from build123d import *

# Parameters (mm, degrees)
BOSS_EXTRUDE1_DEPTH      = 6.35
FILLET1_R                = 12.7
CUT_EXTRUDE2_DEPTH       = 3.175
BOSS_EXTRUDE2_DEPTH      = 3.175
BOSS_EXTRUDE2_DEPTH_BACK = 36.135303
SKETCH4_R                = 9.525
SKETCH4_R_2              = 6.35
SKETCH5_R                = 9.525
SKETCH5_R_2              = 6.35
BOSS_EXTRUDE3_DEPTH      = 25.4
CHAMFER2_SIZE            = 1


with BuildPart() as part:
    # Sketch1 → Boss-Extrude1 (new, symmetric)
    with BuildSketch(Plane.YZ):
        Polygon((-25.4, 10.735303163), (0, 25.4), (25.4, 25.4), (25.4, -25.4), (-25.4, -25.4), align=None)
    extrude(amount=BOSS_EXTRUDE1_DEPTH, both=True)

    # Fillet1
    fillet1_edges = [part.edges().sort_by_distance(p)[0] for p in [
        (0, 25.4, -25.4),
    ]]
    fillet(fillet1_edges, radius=FILLET1_R)

    # Sketch3 → Cut-Extrude2 (cut)
    with BuildSketch(Plane.YZ.offset(6.35)):
        with BuildLine():
            Line((-22.225, -22.225), (12.7, -22.225))
            ThreePointArc((12.7, -22.225), (19.435192091, -19.435192091), (22.225, -12.7))
            Line((22.225, -12.7), (22.225, 22.225))
            Line((22.225, 22.225), (0.850738686, 22.225))
            Line((0.850738686, 22.225), (-22.225, 8.902216058))
            Line((-22.225, 8.902216058), (-22.225, -22.225))
        make_face()
    cut_extrude2 = extrude(amount=-CUT_EXTRUDE2_DEPTH, mode=Mode.SUBTRACT)

    # Mirror1: Cut-Extrude2 across plane
    add(cut_extrude2.mirror(Plane(origin=(0, 0, 0), x_dir=(0, 0, 1), z_dir=(1, 0, 0))), mode=Mode.SUBTRACT)

    # Sketch4 → Boss-Extrude2 (add, two sides: drawn at the far end of the back side and taken through both)
    with BuildSketch(Plane(origin=(0, 0, -25.4), x_dir=(1, 0, 0), z_dir=(0, 0, -1)).offset(-BOSS_EXTRUDE2_DEPTH_BACK)):
        with Locations(Location((0, 33.02, 0), (0, 0, 233.130102354))):
            Circle(SKETCH4_R)
        with Locations(Location((0, 33.02, 0), (0, 0, 270))):
            Circle(SKETCH4_R_2, mode=Mode.SUBTRACT)
    extrude(amount=BOSS_EXTRUDE2_DEPTH + BOSS_EXTRUDE2_DEPTH_BACK)

    # Sketch5 → Boss-Extrude3 (add)
    with BuildSketch(Plane(origin=(0, 25.4, 0), x_dir=(-1, 0, 0), z_dir=(0, 1, 0))):
        with Locations((0, 33.02)):
            Circle(SKETCH5_R)
        with Locations(Location((0, 33.02, 0), (0, 0, 90))):
            Circle(SKETCH5_R_2, mode=Mode.SUBTRACT)
    extrude(amount=-BOSS_EXTRUDE3_DEPTH)

    # Chamfer2
    # the kernel refuses this chamfer: 1 mm, written as the material it takes off along each edge
    with BuildSketch(Plane(origin=(0, -33.02, 10.735303), x_dir=(0.3638595085405839, 0.931453841070294, 0), z_dir=(-0.931453841070294, 0.3638595085405839, 0))) as chamfer2_piece_1_section:
        Polygon((9.525, CHAMFER2_SIZE), (9.525 - CHAMFER2_SIZE, 0), (9.525, 0), align=None)
    chamfer2_piece_1 = revolve(axis=Axis((0, -33.02, 10.735303), (0, 0, -1)), revolution_arc=317.325176487, mode=Mode.PRIVATE)
    chamfer2_piece_1 = split(chamfer2_piece_1, bisect_by=Plane(origin=(5.777045626, -25.4, 10.24862198), z_dir=(0, -1, 0)), keep=Keep.TOP, mode=Mode.PRIVATE)
    add(chamfer2_piece_1, mode=Mode.SUBTRACT)
    with BuildSketch(Plane(origin=(0, -33.02, -28.575), x_dir=(-0.6000000000021781, 0.7999999999983665, 0), z_dir=(-0.7999999999983665, -0.6000000000021781, 0))) as chamfer2_piece_2:
        Polygon((9.525, -CHAMFER2_SIZE), (9.525 - CHAMFER2_SIZE, 0), (9.525, 0), align=None)
    revolve(axis=Axis((0, -33.02, -28.575), (0, 0, -1)), mode=Mode.SUBTRACT)
    with BuildSketch(Plane(origin=(0, 25.4, 33.02), x_dir=(-0.3638595085405501, 0, -0.9314538410703074), z_dir=(0.9314538410703074, 0, -0.3638595085405501))) as chamfer2_piece_3_section:
        Polygon((9.525, -CHAMFER2_SIZE), (9.525 - CHAMFER2_SIZE, 0), (9.525, 0), align=None)
    chamfer2_piece_3 = revolve(axis=Axis((0, 25.4, 33.02), (0, 1, 0)), revolution_arc=317.325176487, mode=Mode.PRIVATE)
    chamfer2_piece_3 = split(chamfer2_piece_3, bisect_by=Plane(origin=(0, 24.920234358, 25.4), z_dir=(0, 0, 1)), keep=Keep.TOP, mode=Mode.PRIVATE)
    add(chamfer2_piece_3, mode=Mode.SUBTRACT)
    with BuildSketch(Plane(origin=(0, 0, 33.02), x_dir=(-0.3638595085405531, 0, -0.9314538410703063), z_dir=(0.9314538410703063, 0, -0.3638595085405531))) as chamfer2_piece_4_section:
        Polygon((9.525, CHAMFER2_SIZE), (9.525 - CHAMFER2_SIZE, 0), (9.525, 0), align=None)
    chamfer2_piece_4 = revolve(axis=Axis((0, 0, 33.02), (0, 1, 0)), revolution_arc=317.325176487, mode=Mode.PRIVATE)
    chamfer2_piece_4 = split(chamfer2_piece_4, bisect_by=Plane(origin=(-5.452412952, 0.490850729, 25.4), z_dir=(0, 0, 1)), keep=Keep.TOP, mode=Mode.PRIVATE)
    add(chamfer2_piece_4, mode=Mode.SUBTRACT)

    # Sweep3: sweep along a path in Sketch6
    with BuildLine(Plane.YZ) as sweep3_path:
        Line((0, 33.02), (-20.32, 33.02))
        ThreePointArc((-20.32, 33.02), (-29.300256121, 29.300256121), (-33.02, 20.32))
        Line((-33.02, 20.32), (-33.02, 10.735303163))
    # Sketch7 → Sweep3 (sweep)
    with BuildSketch(Plane.XZ):
        with BuildLine():
            Line((-8.525, 33.02), (-6.35, 33.02))
            ThreePointArc((-6.35, 33.02), (0, 26.67), (6.35, 33.02))
            Line((6.35, 33.02), (8.525, 33.02))
            ThreePointArc((8.525, 33.02), (0, 24.495), (-8.525, 33.02))
        make_face()
    sweep(path=sweep3_path.line)


solid = part.part
Design review of the part built by this model. Coordinates are the model's own, in mm. A direction names the side the tool comes from. Round coordinates to 2 decimals unless told otherwise and drop trailing zeros. Loops run counter-clockwise (first coordinate to the right, second up) from the corner with the lowest first, then second, coordinate; pieces in that order, holes last. Notation, with made-up numbers: M 67.5,62.25 L 94.5,62.25 A17 cw 94.5,70.25 Z; hole C -32,51.25 d1. An arc over 180 degrees is marked long. Answer as a JSON object with one key per item and string values.
Item 1: The part is to be moulded in two halves that separate along Z. For faces 1 (the cylindrical face through (0.09, 21.58, -21.78)), 2 (the flat face through (3.175, 0, 0)), 3 (the flat face through (-3.175, 0, 0)), 4 (the flat face through (-6.35, -9, 17)), say which applies: pulls with the +Z half, pulls with the -Z half, needs draft (parallel to the pull), parting line crosses it, or undercut.
Answer sheet:
{"face 1": "pulls with the -Z half", "face 2": "undercut", "face 3": "undercut", "face 4": "needs draft"}
Item 2: We need section C-C on y = -4. Give the boundary of the cut face in (x, z) (3 decimals), and give its area (3 significant figures).
Answer sheet:
{"outline": "M -8.525,33.02 A8.525 ccw 8.525,33.02 L 6.35,33.02 A6.35 cw -6.35,33.02 Z; M -6.35,-25.4 L 6.35,-25.4 L 6.35,-22.225 L 3.175,-22.225 L 3.175,19.424 L 6.35,19.424 L 6.35,23.091 L -6.35,23.091 L -6.35,19.424 L -3.175,19.424 L -3.175,-22.225 L -6.35,-22.225 Z", "area": "402 mm^2"}
Item 3: Wall thickness on L1, parallel to X at y = 5, z = 33; L2, parallel to Y at x = -3.5, z = -9.5 (3 decimals); L3, parallel to Z at x = 0, y = 8.25 (3 decimals): over which ranges is each line inside the solid? List them lowest first. Write a range as from..to.
Answer sheet:
{"L1": "x = -9.52..-6.35, 6.35..9.52", "L2": "y = -41.879..-38.318, -27.722..-22.225, 22.225..25.4", "L3": "z = -25.4..26.67, 39.37..42.545"}
Item 4: Machinability: for faces 5 (the flat face through (-5, 22.225, 5)), 6 (the flat face through (7, -33.02, 15)), 7 (the conical face through (0.325, -41.699, 10.576)), 8 (the flat face through (5, 22.225, 5)), 9 (the flat face through (6, -30, -28.575)), which of the approach directions +Z, -Z, +X, -X, +Y, -Y give a long, thin tool a straight path to every point of the face, cutting with its end or side? Answer none if there is none.
Answer sheet:
{"face 5": "-X", "face 6": "+Z, +X, -X, -Y", "face 7": "none", "face 8": "+X", "face 9": "-Z, +X, -X, +Y, -Y"}
Item 5: We need section D-D on y = 8. Give the boundary of the cut face in (x, z) (3 decimals).
Answer sheet:
{"outline": "M -6.35,-25.4 L 6.35,-25.4 L 6.35,-22.225 L 3.175,-22.225 L 3.175,22.225 L 6.35,22.225 L 6.35,25.4 L 5.715,25.4 A9.525 ccw long -5.715,25.4 L -6.35,25.4 L -6.35,22.225 L -3.175,22.225 L -3.175,-22.225 L -6.35,-22.225 Z; hole C 0,33.02 d12.7"}
Item 6: We need section B-B on x = 0. State how many separate pieces and enclosed holes the cut face has, and give its area (3 significant figures).
Answer sheet:
{"separate pieces": "3", "enclosed holes": "1", "area": "2,730 mm^2"}
Item 7: We need section A-A on z = 14.5. Give the boundary of the cut face in (x, y) (3 decimals).
Answer sheet:
{"outline": "M -8.525,-33.02 L -6.35,-33.02 A6.35 cw 6.35,-33.02 L 8.525,-33.02 A8.525 ccw Z; M -6.35,-18.879 L 6.35,-18.879 L 6.35,-12.529 L 3.175,-12.529 L 3.175,22.225 L 6.35,22.225 L 6.35,25.4 L -6.35,25.4 L -6.35,22.225 L -3.175,22.225 L -3.175,-12.529 L -6.35,-12.529 Z"}
Item 8: Clearance check with flat-ended pins moving along their axes: P1, Ø5, axis at y = 10.5, z = 21.5, coming from the +X side; P2, Ø1, axis at x = -2, y = -9, coming from the +Z side; P3, Ø5, axis at y = 1.5, z = 10, coming from the -X side (3 decimals); P4, Ø4, axis at x = -4, y = -29, coming from the -Z side (3 decimals). State where each tip first meets the part, or that it passes through.
Answer sheet:
{"P1": "stops at x = 6.35", "P2": "stops at z = 27.18", "P3": "stops at x = -3.175", "P4": "stops at z = -28.575"}
